Can you work these out from the model? Positions are in its coordinate system, mm. Face numbers are marked on the shaded views. A direction names the side the tool comes from. Round coordinates to 2 decimals unless told otherwise and drop trailing zeros. Loops run counter-clockwise (first coordinate to the right, second up) from the corner with the lowest first, then second, coordinate; pieces in that order, holes last. Notation, with made-up numbers: (60, 41.5) -> (113, 41.5) arc R20 cw to (113, 46.5) -> close; hole circle Ø4 at (-26, -37). An arc over 180 degrees is marked (long way). Write item = value, one per line.
from build123d import *

# Parameters (mm, degrees)
SKETCH_W          = 25
SKETCH_H          = 11
SKETCH_R          = 1.6
PAD_DEPTH         = 4
POCKET_DEPTH      = 18
SKETCH002_W       = 5
SKETCH002_H       = 3.25
PAD001_DEPTH      = 2
SKETCH003_W       = 3
SKETCH003_H       = 11
PAD002_DEPTH      = 4
PAD002_DEPTH_BACK = 8
SKETCH004_R       = 1.45
POCKET001_DEPTH   = 25.001


with BuildPart() as part:
    # Sketch → Pad (new body)
    with BuildSketch(Plane.XY):
        with Locations((12.5, 5.5)):
            Rectangle(SKETCH_W, SKETCH_H)
        with Locations((22, 8)):
            Circle(SKETCH_R, mode=Mode.SUBTRACT)
    extrude(amount=PAD_DEPTH)

    # Sketch001 → Pocket (cut)
    with BuildSketch(Plane.YZ):
        Polygon((1, 3), (7, 3), (7, 1.5), (6, 1.5), (6, 0), (2, 0), (2, 1.5), (1, 1.5), align=None)
    extrude(amount=POCKET_DEPTH, mode=Mode.SUBTRACT)

    # Sketch002 (on DatumPlane) → Pad001 (join)
    with BuildSketch(Plane.XY.offset(4)):
        with Locations((2.5, 1.625)):
            Rectangle(SKETCH002_W, SKETCH002_H)
    extrude(amount=PAD001_DEPTH)

    # Sketch003 → Pad002 (join, two sides)
    with BuildSketch(Plane.XY) as pad002_sk:
        with Locations((17, 5.5)):
            Rectangle(SKETCH003_W, SKETCH003_H)
    extrude(amount=PAD002_DEPTH)
    extrude(pad002_sk.sketch, amount=-PAD002_DEPTH_BACK)

    # Sketch004 → Pocket001 (cut, through all)
    with BuildSketch(Plane.YZ):
        with Locations((4, -4)):
            Circle(SKETCH004_R)
    extrude(amount=POCKET001_DEPTH, mode=Mode.SUBTRACT)


solid = part.part
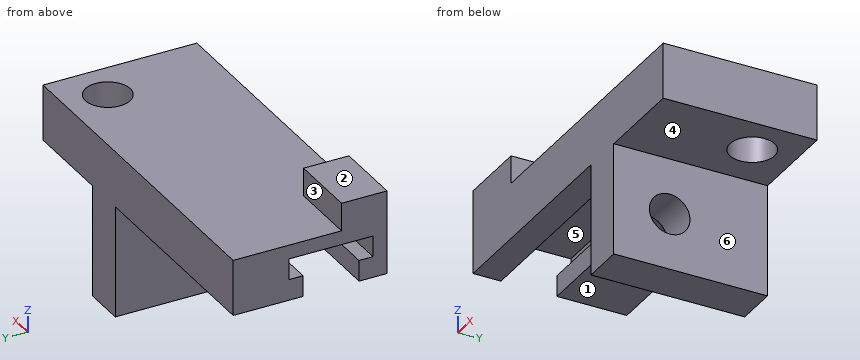
1. Suppose I cut it at C-C, the plane x = 22. List the corners of the cut face in (y, z) for me.
Entries:
outline = (0, 0) -> (6.4, 0) -> (6.4, 4) -> (0, 4) -> close; (9.6, 0) -> (11, 0) -> (11, 4) -> (9.6, 4) -> close
2. We'd pull the mould along Z, two halves only. Please class the marked faces 4, 5 and 6: released by +Z, released by -Z, zero draft, split by the parting line, or undercut.
Entries:
face_4 = released by -Z
face_5 = undercut
face_6 = zero draft
3. I'm going to push flat-ended pins straight in: pin 1 (0.5 mm diameter, centred on x = 9.5, y = 6.5, fed in from +Z); pin 2 (2.5 mm diameter, centred on y = 4, z = -4, fed in from +X); pin 3 (2 mm diameter, centred on x = 22.5, y = 5, fed in from -Z); pin 4 (2.5 mm diameter, centred on y = 8, z = -3, fed in from +X). Where does each tip first touch, or does it pass through?
Entries:
pin_1 = 4
pin_2 = through
pin_3 = 0
pin_4 = 18.5
4. For the marked faces 1, 2 and 3, which set-ups out of +Z, -Z, +X, -X, +Y, -Y let a thin tool reach every point of the face, with its end or its side?
Entries:
face_1 = -Z, -X, +Y, -Y
face_2 = +Z, +X, -X, +Y, -Y
face_3 = +Z, +X, -X, +Y
5. Suppose I cut it at D-D, the plane x = 12.5. List the corners of the cut face in (y, z) for me, and give its area (3 significant figures).
Entries:
outline = (0, 0) -> (2, 0) -> (2, 1.5) -> (1, 1.5) -> (1, 3) -> (7, 3) -> (7, 1.5) -> (6, 1.5) -> (6, 0) -> (11, 0) -> (11, 4) -> (0, 4) -> close
area = 29.0 mm²
6. I need wall thicknesses on line 1 (Z direction, x = 14.5, y = 6.25); line 2 (Z direction, x = 16.4, y = 4); line 3 (Y direction, x = 7, z = 1.25). Which ranges of each line are inside material? Lowest first, please. Write a range as [from, to].
Entries:
line_1 = [0, 1.5], [3, 4]
line_2 = [-8, -5.45], [-2.55, 4]
line_3 = [0, 2], [6, 11]
7. Suppose I cut it at A-A, the plane y = 4. List the corners of the cut face in (x, z) for me, and give its area (3 significant figures).
Entries:
outline = (0, 3) -> (15.5, 3) -> (15.5, -2.55) -> (18.5, -2.55) -> (18.5, 0) -> (25, 0) -> (25, 4) -> (0, 4) -> close; (15.5, -8) -> (18.5, -8) -> (18.5, -5.45) -> (15.5, -5.45) -> close
area = 68.8 mm²
8. Suppose I cut it at B-B, the plane z = -4. List the corners of the cut face in (x, y) for me, and give its area (3 significant figures).
Entries:
outline = (15.5, 0) -> (18.5, 0) -> (18.5, 2.55) -> (15.5, 2.55) -> close; (15.5, 5.45) -> (18.5, 5.45) -> (18.5, 11) -> (15.5, 11) -> close
area = 24.3 mm²
